```python
from build123d import *

# Parameters (mm, degrees)
BOSS_EXTRUDE2_DEPTH     = 30
SKETCH3_R               = 3
CUT_EXTRUDE1_DEPTH      = 30
FILLET7_R               = 15
FILLET8_R               = 15
CUT_EXTRUDE2_DEPTH      = 30
CUT_EXTRUDE2_DEPTH_BACK = 30
SKETCH6_R               = 3
SKETCH7_W               = 10
SKETCH7_H               = 10.288497565
BOSS_EXTRUDE3_DEPTH     = 19.923787886
SKETCH8_R               = 3
CUT_EXTRUDE3_DEPTH      = 10
FILLET12_R              = 5
FILLET15_R              = 5.3
FILLET17_R              = 15
SKETCH9_W               = 1.5
SKETCH9_H               = 30
CUT_EXTRUDE4_DEPTH      = 15.39622199


# Some blends are built 0.0001 mm under size
with BuildPart() as part:
    # Sketch2 → Boss-Extrude2 (new body)
    with BuildSketch(Plane(origin=(0, 0, 0), x_dir=(1, 0, 0), z_dir=(0, 1, 0))):
        Polygon((0, 0), (14.595501533, 0), (14.595501533, 35), (4.595501533, 35), (4.595501533, 25.288497565), (-5.404498467, 25.288497565), (-5.404498467, 35), (-15.404498467, 35), (-15.404498467, 15), (0, 15), align=None)
    extrude(amount=BOSS_EXTRUDE2_DEPTH)

    # Sketch3 → Cut-Extrude1 (cut)
    with BuildSketch(Plane.ZY):
        with Locations((-7.5, 15)):
            Circle(SKETCH3_R)
    extrude(amount=-CUT_EXTRUDE1_DEPTH, mode=Mode.SUBTRACT)

    # Fillet7
    fillet7_edges = [part.edges().sort_by_distance(p)[0] for p in [
        (7.297750767, 30, 0),
    ]]
    fillet(fillet7_edges, radius=FILLET7_R)

    # Fillet8
    fillet8_edges = [part.edges().sort_by_distance(p)[0] for p in [
        (7.297750767, 0, 0),
    ]]
    fillet(fillet8_edges, radius=FILLET8_R - 0.0001)  # a hair under: the kernel refuses the full size

    # Sketch6 → Cut-Extrude2 (cut, two sides: drawn at the far end of the back side and taken through both)
    with BuildSketch(Plane.ZY.offset(-4.595501533).offset(-CUT_EXTRUDE2_DEPTH_BACK)):
        with Locations(Location((-28.393945452, 15, 0), (0, 0, 180))):
            Circle(SKETCH6_R)
    extrude(amount=CUT_EXTRUDE2_DEPTH + CUT_EXTRUDE2_DEPTH_BACK, mode=Mode.SUBTRACT)

    # Sketch7 → Boss-Extrude3 (add)
    with BuildSketch(Plane(origin=(0, 30, 0), x_dir=(1, 0, 0), z_dir=(0, 1, 0))):
        with Locations((-0.404498467, 20.144248783)):
            Rectangle(SKETCH7_W, SKETCH7_H)
    extrude(amount=BOSS_EXTRUDE3_DEPTH)

    # Sketch8 → Cut-Extrude3 (cut)
    with BuildSketch(Plane(origin=(4.595501533, 0, 0), x_dir=(0, 0, -1), z_dir=(1, 0, 0))):
        with Locations((20.144248782, 41.414541631)):
            Circle(SKETCH8_R)
    extrude(amount=-CUT_EXTRUDE3_DEPTH, mode=Mode.SUBTRACT)

    # Fillet12
    fillet12_edges = [part.edges().sort_by_distance(p)[0] for p in [
        (-0.404498467, 49.923787886, -15),
    ]]
    fillet(fillet12_edges, radius=FILLET12_R)

    # Fillet15
    # the kernel refuses this fillet: 5.3 mm, written as the material it takes off along each edge
    with BuildSketch(Plane(origin=(17.845501533, 49.923787886, -25.288497565), x_dir=(0, 0, 1), z_dir=(-1, 0, 0))) as fillet15_piece_1:
        with BuildLine():
            CenterArc((FILLET15_R, -FILLET15_R), FILLET15_R, 90, 90)
            Line((0, -FILLET15_R), (-FILLET15_R * 0.02, -FILLET15_R))
            Line((-FILLET15_R * 0.02, -FILLET15_R), (-FILLET15_R * 0.02, FILLET15_R * 0.02))
            Line((-FILLET15_R * 0.02, FILLET15_R * 0.02), (FILLET15_R, FILLET15_R * 0.02))
            Line((FILLET15_R, FILLET15_R * 0.02), (FILLET15_R, 0))
        make_face()
    extrude(amount=36.5, mode=Mode.SUBTRACT)

    # Fillet17
    # the kernel refuses this fillet: 15 mm, written as the material it takes off along each edge
    with BuildSketch(Plane(origin=(52.095501533, 30, -35), x_dir=(0, 0, 1), z_dir=(-1, 0, 0)), Plane(origin=(-5.404498467, 30, -35), x_dir=(0, 0, 1), z_dir=(-1, 0, 0))) as fillet17_piece_1:
        with BuildLine():
            CenterArc((FILLET17_R, -FILLET17_R), FILLET17_R, 90, 90)
            Line((0, -FILLET17_R), (0, 0))
            Line((0, 0), (FILLET17_R, 0))
        make_face()
    extrude(amount=47.5, mode=Mode.SUBTRACT)
    with BuildSketch(Plane(origin=(52.095501533, 30, -35), x_dir=(0, 0, 1), z_dir=(-1, 0, 0))) as fillet17_piece_2_section:
        with BuildLine():
            CenterArc((FILLET17_R, -FILLET17_R), FILLET17_R, 90, 90)
            Line((0, -FILLET17_R), (0, 0))
            Line((0, 0), (FILLET17_R, 0))
        make_face()
    fillet17_piece_2 = extrude(amount=85, mode=Mode.PRIVATE)
    fillet17_piece_2 = split(fillet17_piece_2, bisect_by=Plane(origin=(-5.404498467, 29.712703536, -23.975011992), z_dir=(-1, 0, 0)), keep=Keep.TOP, mode=Mode.PRIVATE)
    add(fillet17_piece_2, mode=Mode.SUBTRACT)
    with BuildSketch(Plane(origin=(32.095501533, 0, -35), x_dir=(0, 0, 1), z_dir=(-1, 0, 0))) as fillet17_piece_3:
        with BuildLine():
            CenterArc((FILLET17_R, FILLET17_R), FILLET17_R, 180, 90)
            Line((0, FILLET17_R), (0, 0))
            Line((0, 0), (FILLET17_R, 0))
        make_face()
    extrude(amount=85, mode=Mode.SUBTRACT)
    with BuildSketch(Plane(origin=(32.095501533, 30, -35), x_dir=(0, 0, 1), z_dir=(-1, 0, 0))) as fillet17_piece_4_section:
        with BuildLine():
            CenterArc((FILLET17_R, -FILLET17_R), FILLET17_R, 90, 90)
            Line((0, -FILLET17_R), (0, 0))
            Line((0, 0), (FILLET17_R, 0))
        make_face()
    fillet17_piece_4 = extrude(amount=85, mode=Mode.PRIVATE)
    fillet17_piece_4 = split(fillet17_piece_4, bisect_by=Plane(origin=(4.595501533, 29.712703536, -23.975011992), z_dir=(1, 0, 0)), keep=Keep.TOP, mode=Mode.PRIVATE)
    add(fillet17_piece_4, mode=Mode.SUBTRACT)

    # Sketch9 → Cut-Extrude4 (cut)
    with BuildSketch(Plane.ZY.offset(15.404498467)):
        with Locations((-15.75, 15)):
            Rectangle(SKETCH9_W, SKETCH9_H)
    extrude(amount=-CUT_EXTRUDE4_DEPTH, mode=Mode.SUBTRACT)


solid = part.part
```
Source: CAD feature listing. Evaluate the final solid. Frame: model axes, mm. A direction names the side the tool comes from. Give positions to 0.01 mm unless a question says otherwise; leave off trailing zeros. Loops run counter-clockwise (first coordinate to the right, second up) from the corner with the lowest first, then second, coordinate; pieces in that order, holes last. Notation, with made-up numbers: (-6.75, 42) -> (52.25, 42) arc R14 cw to (52.25, 49) -> close; hole circle Ø3 at (-20.5, -32). An arc over 180 degrees is marked (long way). Put each result on its own line as item: value. Start each with the question number.
1) Cut plane A-A (y = 16.5). State how many separate pieces and enclosed holes the cut face has, then the cut area to 3 significant figures.
2) Material intervals for probe 1 along X at (y, z) = (21, -32); probe 2 along Z at (x, y) = (-5, 4); probe 3 along X at (y, z) = (14, -13), sorted ascending.
3) Draft query along X for faces 6 (the face through (4.596, 15, -32)), 7 (the face through (-10, 30, -18)), 8 (the face through (-0.008, 15, -16)). Return one class per face: released by +X, released by -X, zero draft, split by the parting line, or undercut.
4) Cut plane D-D (z = -18). Return loops of the section in (x, y), then the cut area to 3 significant figures.
5) Contact query for flat-ended pins moving along their axis: P1, Ø4, axis at x = 12, z = -17.5, coming from the +Y side; P2, Ø1.5, axis at x = -3, y = 21.5, coming from the +Z side; P3, Ø0.8, axis at y = 17, z = -16, coming from the -X side. Output: stop coordinate, or through.
6) Cut plane C-C (z = -26). Return loops of the section in (x, y), then the cut area to 3 significant figures.
7) Reachability of faces 1 (the face through (0, 15, -11)), 2 (the face through (-5.404, 15, -32)), 3 (the face through (-3, 30, -16)), 4 (the face through (7.4, 25.49, -4.28)), 5 (the face through (10, 30, -18)) from +Z, -Z, +X, -X, +Y, -Y: full face, straight path, thin tool, end or side. Return the list, or none.
Results are:
1. separate pieces: 4
1. enclosed holes: 0
1. area: 516 mm2
2. probe 1: x = -15.4 to -5.4, 4.6 to 14.6
2. probe 2: z = -25.29 to -16.5
2. probe 3: x = 0 to 14.6
3. face 6: undercut
3. face 7: zero draft
3. face 8: released by -X
4. outline: (-15.4, 0) -> (14.6, 0) -> (14.6, 30) -> (4.6, 30) -> (4.6, 39.32) -> (-5.4, 39.32) -> (-5.4, 30) -> (-15.4, 30) -> close; (-5.4, 43.51) -> (4.6, 43.51) -> (4.6, 49.51) -> (-5.4, 49.51) -> close
4. area: 1,050 mm2
5. P1: stops at y = 30
5. P2: stops at z = -16.5
5. P3: stops at x = -0.01
6. outline: (-15.4, 1.25) -> (-5.4, 1.25) -> (-5.4, 13.19) -> (-15.4, 13.19) -> close; (-15.4, 16.81) -> (-5.4, 16.81) -> (-5.4, 28.75) -> (-15.4, 28.75) -> close; (4.6, 1.25) -> (14.6, 1.25) -> (14.6, 13.19) -> (4.6, 13.19) -> close; (4.6, 16.81) -> (14.6, 16.81) -> (14.6, 28.75) -> (4.6, 28.75) -> close
6. area: 478 mm2
7. face 1: +Z, -X, +Y, -Y
7. face 2: -Z, +Y, -Y
7. face 3: +Z, -X, -Y
7. face 4: +Z, +X, -X, +Y
7. face 5: +Z, -Z, +X, +Y
